Here's how the part is built. I have some questions about the finished solid (model axes, mm). A direction names the side the tool comes from. Coordinates: 2 decimals unless noted, no trailing zeros. Write each loop counter-clockwise with the first axis right and the second up, starting at its lowest first coordinate (ties: lowest second). Pieces come first, ordered by that corner, then holes.
(1) Imagine slicing it at A-A, the plane x = -0.5. List the corners of the cut face in (y, z) for me, plus the area to 3 significant figures.
(2) Which directions (+Z, -Z, +X, -X, +Y, -Y) give clear straight access to the entire face, cutting with the end or side of a thin tool? Please do faces 1 (the flat face through (-1.5, 1, 0)), 2 (the flat face through (3, 1.3, 1.9)), 3 (the flat face through (3, -1.3, 1.9)), 4 (the flat face through (0, 1.3, 1.9)).
(3) For pin 1 Ø1.1 at (y, z) = (-1.5, -2) entering from +X; pin 2 Ø0.5 at (y, z) = (-1.5, -2) entering from -X; pin 3 Ø3 at (y, z) = (-0.5, 2.5) entering from +X, each with a flat end and sliding along its axis, tell me the tip position at first contact or that it passes through.
(4) Imagine slicing it at B-B, the plane y = 1.55. State how many separate pieces and enclosed holes the cut face has, plus the area to 3 significant figures.
(5) Thinking about a two-plate mould opening in Z: for faces 5 (the cylindrical face through (1.48, -0.36, 2.47)), 6 (the flat face through (3, 2.3, 0.7)), which applies, released by +Z, released by -Z, zero draft, split by the parting line, or undercut?
(6) Please list where these lines run through material, in increasing order: probe 1 along Y at (x, z) = (-1.1, 0); probe 2 along Y at (x, z) = (2, 0.8); probe 3 along Y at (x, z) = (3.5, 0).
```python
from build123d import *
from build123d.topology import SkipClean

# Parameters (mm, degrees)
BASPROSKE_W         = 3
BASPROSKE_H         = 3
TOOTHCUT_DEPTH      = 6.196152423
TEETHCUTS_COUNT     = 10
TEETHCUTS_ANGLE     = 324
BORSKE_R            = 0.5
BORE_DEPTH          = 50.0000508
SKETCH_1_R          = 1.874
SKETCH_1_R_2        = 0.5
EXTRUDE_1_DEPTH     = 1.5
FILLET_2_R          = 1.3
EXTRUDE_START       = 3
SKETCH_2_R          = 1.874
SKETCH_2_R_2        = 0.5
EXTRUDE_2_DEPTH     = 3
SKETCH_3_W          = 1
SKETCH_3_H          = 3.761306816
CUT_EXTRUDE_1_DEPTH = 1.5


with BuildPart() as part:
    # BasProSke → Base-Revolve (revolve)
    with BuildSketch(Plane(origin=(0, 0, 0), x_dir=(1, 0, 0), z_dir=(0, 1, 0)), mode=Mode.PRIVATE) as base_revolve_sk:
        with Locations((1.5, 1.5)):
            Rectangle(BASPROSKE_W, BASPROSKE_H)
    revolve(base_revolve_sk.sketch.rotate(Axis((-10, 0, 0), (1, 0, 0)), 180), axis=Axis((-10, 0, 0), (1, 0, 0)))

    # TooCutSke → ToothCut (cut, through all)
    with BuildSketch(Plane(origin=(0, 0, 0), x_dir=(0, 0, -1), z_dir=(1, 0, 0))):
        with BuildLine():
            ThreePointArc((0.296449938, 1.850403587), (0, 1.874), (-0.296449938, 1.850403587))
            ThreePointArc((-0.296449938, 1.850403587), (-0.428089565, 2.470295585), (-0.905889751, 2.886591228))
            ThreePointArc((-0.905889751, 2.886591228), (0, 3.0254), (0.905889751, 2.886591228))
            ThreePointArc((0.905889751, 2.886591228), (0.428089565, 2.470295585), (0.296449938, 1.850403587))
        make_face()
    toothcut = extrude(amount=TOOTHCUT_DEPTH, mode=Mode.SUBTRACT)

    # TeethCuts: ToothCut ×10 about axis
    teethcuts_axis = Axis((-10, 0, 0), (1, 0, 0))
    for i in range(1, TEETHCUTS_COUNT):
        add(toothcut.rotate(teethcuts_axis, i * TEETHCUTS_ANGLE / (TEETHCUTS_COUNT - 1)), mode=Mode.SUBTRACT)

    # BorSke → Bore (cut, symmetric)
    with BuildSketch(Plane(origin=(0, 0, 0), x_dir=(0, 0, -1), z_dir=(1, 0, 0))):
        with Locations(Location((0, 0, 0), (0, 0, 180))):
            Circle(BORSKE_R)
    extrude(amount=BORE_DEPTH, both=True, mode=Mode.SUBTRACT)

    # 草图1 → 凸台-拉伸1 (add)
    with SkipClean():  # the faces are left unmerged after this step: merging them gives an invalid solid
        with BuildSketch(Plane(origin=(3, 0, 0), x_dir=(0, 0, -1), z_dir=(1, 0, 0))):
            with Locations(Location((0, 0, 0), (0, 0, 171.101911086))):
                Circle(SKETCH_1_R)
            Circle(SKETCH_1_R_2, mode=Mode.SUBTRACT)
        extrude(amount=EXTRUDE_1_DEPTH)
    add(part.part.scale(1), mode=Mode.REPLACE)  # the faces are merged on a copy

    # 圆角2
    fillet_2_edges = [part.edges().sort_by_distance(p)[0] for p in [
        (4.5, -0.28986551, -1.851446458),
    ]]
    fillet(fillet_2_edges, radius=FILLET_2_R)

    # 草图2 → 凸台-拉伸2 (add)
    with BuildSketch(Plane.ZY.offset(EXTRUDE_START)):
        Circle(SKETCH_2_R)
        Circle(SKETCH_2_R_2, mode=Mode.SUBTRACT)
    extrude(amount=-EXTRUDE_2_DEPTH)

    # 草图3 → 切除-拉伸1 (cut)
    with BuildSketch(Plane.ZY.offset(3)):
        Rectangle(SKETCH_3_W, SKETCH_3_H)
    extrude(amount=-CUT_EXTRUDE_1_DEPTH, mode=Mode.SUBTRACT)


solid = part.part
```
Recorded:
1. outline: circle Ø3.75 at (0, 0); hole circle Ø1 at (0, 0)
1. area: 10.2 mm2
2. face 1: -X, +Y, -Y
2. face 2: +Z, +X, +Y
2. face 3: +Z, +X, -Y
2. face 4: +Z, -X, +Y
3. pin 1: stops at x = 3
3. pin 2: stops at x = 0
3. pin 3: stops at x = 4.41
4. separate pieces: 3
4. enclosed holes: 0
4. area: 18.5 mm2
5. face 5: undercut
5. face 6: zero draft
6. probe 1: y = -1.87 to -0.5, 0.5 to 1.87
6. probe 2: y = -2.84 to 2.84
6. probe 3: y = -1.84 to -0.5, 0.5 to 1.84
